from build123d import *

# Parameters (mm, degrees)
EXTRUDE_2_DEPTH     = 5
EXTRUDE_3_DEPTH     = 1
EXTRUDE_4_DEPTH     = 1
CUT_EXTRUDE_1_DEPTH = 36.801015056
SKETCH_14_W         = 27.70005588
SKETCH_14_H         = 1.6
CUT_EXTRUDE_2_DEPTH = 6
EXTRUDE_7_DEPTH     = 94.1
SKETCH_16_W         = 32
SKETCH_16_H         = 4.6
EXTRUDE_8_DEPTH     = 2
SKETCH_18_W         = 0.9
SKETCH_18_H         = 1
EXTRUDE_10_DEPTH    = 3.36
FILLET_2_R          = 1


with BuildPart() as part:
    # 草图10 → 凸台-拉伸2 (new body)
    with BuildSketch(Plane.XY):
        Polygon((-0.85513843, -3), (29.14486157, -3), (29.14486157, 9.5), (17.247172974, 9.5), (17.247172974, 17), (-0.85513843, 17), align=None)
        Polygon((0.14486157, 1.6), (0.14486157, 13), (16.247172974, 13), (16.247172974, 4.96), (26.583063246, 4.96), (26.583063246, 1.6), align=None, mode=Mode.SUBTRACT)
    extrude(amount=EXTRUDE_2_DEPTH)

    # 草图11 → 凸台-拉伸3 (add)
    with BuildSketch(Plane.XY.offset(5)):
        Polygon((-1.85513843, -3), (30.14486157, -3), (30.14486157, 10.5), (18.247172974, 10.5), (18.247172974, 18), (-1.85513843, 18), align=None)
    extrude(amount=EXTRUDE_3_DEPTH)

    # 草图12 → 凸台-拉伸4 (add)
    with BuildSketch(Plane(origin=(0, 0, 0), x_dir=(-1, 0, 0), z_dir=(0, 0, -1))):
        Polygon((0.85513843, -3), (1.85513843, -3), (1.85513843, 18), (-18.247172974, 18), (-18.247172974, 10.5), (-30.14486157, 10.5), (-30.14486157, -3), (-29.14486157, -3), align=None)
    extrude(amount=EXTRUDE_4_DEPTH)

    # 草图13 → 切除-拉伸1 (cut, through all)
    with BuildSketch(Plane.XY.offset(6)):
        Polygon((16.247172974, 4.96), (16.247172974, 13), (0.14486157, 13), (0.14486157, 1.6), (26.583063246, 1.6), (26.583063246, 4.96), align=None)
    extrude(amount=-CUT_EXTRUDE_1_DEPTH, mode=Mode.SUBTRACT)

    # 草图14 → 切除-拉伸2 (cut)
    with BuildSketch(Plane(origin=(0, 0, -1), x_dir=(-1, 0, 0), z_dir=(0, 0, -1))):
        with Locations((-13.75002794, 0.8)):
            Rectangle(SKETCH_14_W, SKETCH_14_H)
    extrude(amount=-CUT_EXTRUDE_2_DEPTH, mode=Mode.SUBTRACT)

    # 草图15 → 凸台-拉伸7 (add)
    with BuildSketch(Plane(origin=(0, 0, -1), x_dir=(-1, 0, 0), z_dir=(0, 0, -1))):
        Polygon((-30.14486157, -3), (1.85513843, -3), (1.85513843, 1.6), (0.1, 1.6), (0.1, 0), (-27.60005588, 0), (-27.60005588, 1.6), (-30.14486157, 1.6), align=None)
    extrude(amount=EXTRUDE_7_DEPTH)

    # 草图16 → 凸台-拉伸8 (add)
    with BuildSketch(Plane(origin=(0, 0, -95.1), x_dir=(-1, 0, 0), z_dir=(0, 0, -1))):
        with Locations((-14.14486157, -0.7)):
            Rectangle(SKETCH_16_W, SKETCH_16_H)
    extrude(amount=EXTRUDE_8_DEPTH)

    # 草图18 → 凸台-拉伸10 (add)
    with BuildSketch(Plane(origin=(0, 1.6, 0), x_dir=(1, 0, 0), z_dir=(0, 1, 0))):
        with Locations((16.697172974, -5.5)):
            Rectangle(SKETCH_18_W, SKETCH_18_H)
    extrude(amount=EXTRUDE_10_DEPTH)

    # 圆角2
    fillet_2_edges = [part.edges().sort_by_distance(p)[0] for p in [
        (17.147172974, 4.96, 5.5),
        (17.147172974, 1.6, 5.5),
        (26.583063246, 1.6, 5.5),
        (26.583063246, 4.96, 2.5),
    ]]
    fillet(fillet_2_edges, radius=FILLET_2_R)


solid = part.part
Geometry check sheet. Reference: the model listing, model coordinates, mm. A direction names the side the tool comes from. Coordinates: 2 decimals unless noted, no trailing zeros. Order: outer loops, then holes, each group sorted by start corner. A loop starts at its lowest first (then second) coordinate and runs counter-clockwise, first axis right, second up. Notation, with made-up numbers: M 25,53.5 L 49,53.5 A30 cw 49,78.5 Z; hole C 74.25,44 d1. An arc over 180 degrees is marked long. Use CSV: the item, a comma, the result in double quotes.
Item 1: Mould release check, pull along X, two halves, no side actions. Record for faces 1 (the flat face through (16.247, 8, 3)), 2 (the flat face through (14, 14, -1)), 3 (the flat face through (0.145, 7, 3)), 4 (the flat face through (-1.855, 0, -48)): pulls with the +X half, pulls with the -X half, needs draft (parallel to the pull), parting line crosses it, or undercut.
Returned:
face 1,"undercut"
face 2,"needs draft"
face 3,"undercut"
face 4,"pulls with the -X half"
Item 2: Thickness scan on line 1 along Z through (x, y) = (17.5, 10.25); line 2 along Z through (x, y) = (17.5, 1.25); line 3 along Y through (x, z) = (5, -62). Record the ranges inside material, lowest first.
Returned:
line 1,"z = -1 to 0, 5 to 6"
line 2,"z = -97.1 to -95.1, 5 to 6"
line 3,"y = -3 to 0"
Item 3: Cross-section at A-A on x = 24.5. Record the cut outline in (y, z).
Returned:
outline,"M -3,-97.1 L 1.6,-97.1 L 1.6,-95.1 L 0,-95.1 L 0,5 L 1.6,5 L 1.6,6 L -3,6 Z; M 4.96,-1 L 10.5,-1 L 10.5,0 L 9.5,0 L 9.5,5 L 10.5,5 L 10.5,6 L 4.96,6 Z"
Item 4: Tool access check on faces 5 (the flat face through (17.247, 13, 2)), 6 (the flat face through (14, 1, 5)), 7 (the flat face through (28, 1.6, -49)), 8 (the flat face through (29.145, 3, 2)), 9 (the flat face through (18, 10, 0)). Record the directions out of +Z, -Z, +X, -X, +Y, -Y that give a thin tool (end or side, any length) a straight path to the whole face; none if there is none.
Returned:
face 5,"+X, +Y"
face 6,"none"
face 7,"-Z, +X, -X, +Y"
face 8,"+X, +Y, -Y"
face 9,"+Y"
Item 5: Gauge pin test, flat ends, axial feed: pin 1 Ø4 at (x, y) = (20.5, 5) entering from -Z; pin 2 Ø1.1 at (x, z) = (25.5, 5.5) entering from +Y; pin 3 Ø2 at (x, z) = (19.5, -6) entering from +Y. Record the tip position at first contact, or that the pin passes through.
Returned:
pin 1,"stops at z = -1"
pin 2,"stops at y = 10.5"
pin 3,"stops at y = 0"
Item 6: Cross-section at C-C on x = 14.5. Record the cut outline in (y, z).
Returned:
outline,"M -3,-97.1 L 1.6,-97.1 L 1.6,-95.1 L 0,-95.1 L 0,5 L 1.6,5 L 1.6,6 L -3,6 Z; M 13,-1 L 18,-1 L 18,0 L 17,0 L 17,5 L 18,5 L 18,6 L 13,6 Z"
Item 7: Cross-section at B-B on z = -15. Record the cut outline in (x, y), then the cut area to 3 significant figures.
Returned:
outline,"M -1.86,-3 L 30.14,-3 L 30.14,1.6 L 27.6,1.6 L 27.6,0 L -0.1,0 L -0.1,1.6 L -1.86,1.6 Z"
area,"103 mm2"
